For this review, take the finished solid that the model builds, in its own axes (mm). Face numbers are marked on the shaded views. A direction names the side the tool comes from. Give positions to 0.01 mm unless a question says otherwise; leave off trailing zeros. Write each loop counter-clockwise with the first axis right and the second up, starting at its lowest first coordinate (ties: lowest second). Pieces come first, ordered by that corner, then holes. Notation, with made-up numbers: M 69,80 L 123,80 A15 ccw 123,103 Z; hole C 42.25,20.5 d1. An arc over 180 degrees is marked long. Write item = value, one per line.
Autodesk Inventor part; units mm, degrees
ref_plane "YZ Plane" through (0, 0, 0) normal (1, 0, 0) x (0, 1, 0)
ref_plane "XZ Plane" through (0, 0, 0) normal (0, 1, 0) x (-1, 0, 0)
ref_plane "XY Plane" through (0, 0, 0) normal (0, 0, 1) x (1, 0, 0)
sketch "Sketch1" plane through (0, 0, 0) normal (0, 0, 1) x (1, 0, 0)
  line L0 (7.35, 0) -> (7.35, 19.8)
  line L1 (7.35, 0) -> (27.15, 0) construction
  line L2 (5.35, 21.8) -> (-5.35, 21.8)
  line L3 (-7.35, 19.8) -> (-7.35, 0)
  line L4 (-7.35, 0) -> (7.35, 0)
  arc A0 (-5.35, 21.8) -> (-7.35, 19.8) centre (-5.35, 19.8) ccw
  arc A1 (7.35, 19.8) -> (5.35, 21.8) centre (5.35, 19.8) ccw
  line L5 (90, 15.1029) -> (90, 0) construction
  point P0 (0, 0)
  point P1 (7.35, 21.8)
  point P2 (-7.35, 21.8)
  point P3 (0, 0)
  dimension "d0" = 21.8
  dimension "d1" = 90
  dimension "d2" = 7.35
  dimension "d3" = 14.7
  dimension "d4" = 2
  dimension "d5" = 90
  dimension "d7" = 0
revolve "Revolution1" add sketch "Sketch1" angle 190 about axis through (90, 15.1029, 0) along (0, -1, 0)
properties part number "InertiaKitInner"
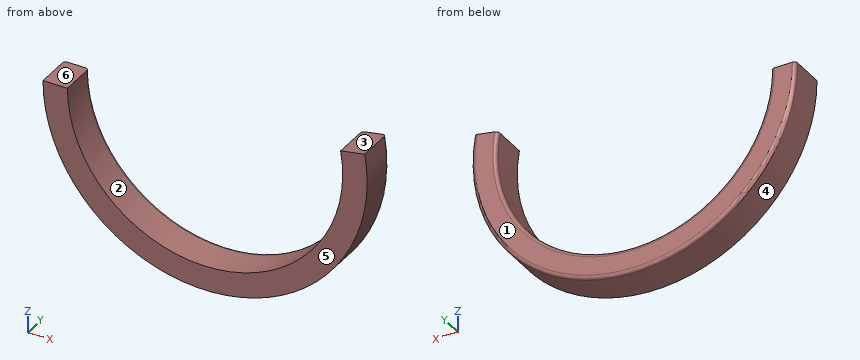
1. Insertion check: P1, Ø12, axis at x = 66.5, y = 9.5, coming from the +Z side; P2, Ø1.5, axis at x = 107.5, y = 5, coming from the +Z side; P3, Ø10, axis at x = 66.5, y = 14.5, coming from the +Z side. Each pin has a flat end and moves straight along its axis. Give the tip position at first contact, or say it passes through.
Responses:
P1 = -77.21
P2 = -80.61
P3 = -77.58
2. Machinability: for the marked faces 5 and 6, which of the approach directions +Z, -Z, +X, -X, +Y, -Y give a long, thin tool a straight path to every point of the face, cutting with its end or side? Answer none if there is none.
Responses:
face_5 = +Z, -Z, +X, -X, -Y
face_6 = +Z, -X, +Y, -Y
3. For line 1 along X through (y, z) = (10, -9.5); line 2 along Z through (x, y) = (91, 3.5); line 3 along X through (y, z) = (16.5, -50.5), list the stretches that pass through material, from the lowest coordinate up. Write a range as from..to.
Responses:
line_1 = -6.89..7.9, 172.1..186.89
line_2 = -97.34..-82.64
line_3 = 6.77..24.57, 155.43..173.23
4. The part is to be moulded in two halves that separate along X. For the marked faces 1, 2, 3 and 4, say which applies: +X half, -X half, draft (parallel to the pull), parting line (faces both ways), or undercut.
Responses:
face_1 = draft
face_2 = undercut
face_3 = -X half
face_4 = parting line
5. We need section A-A, the plane x = 90. Write out the cut boundary in (y, z).
Responses:
outline = M 0,-97.35 L 19.8,-97.35 A2 ccw 21.8,-95.35 L 21.8,-84.65 A2 ccw 19.8,-82.65 L 0,-82.65 Z
6. We need section B-B, the plane y = 8. Write out the cut boundary in (x, z), then the cut area to 3 significant figures.
Responses:
outline = M -7.35,0 A97.35 ccw long 185.87,16.9 L 171.39,14.35 A82.65 cw long 7.35,0 Z
area = 4,390 mm2
